from build123d import *

# Parameters (mm, degrees)
F1_DEPTH = 30
F0_W     = 30
F0_H     = 61.715728
F2_DEPTH = 60


with BuildPart() as f1:
    # F0 (on Front) → F1 (new body)
    with BuildSketch(Plane.XZ):
        with BuildLine():
            Line((-168.30257, -116.075176), (-168.30257, -201.93304))
            ThreePointArc((-168.30257, -201.93304), (-174.475736, -211.171836), (-185.373638, -209.004108))
            Line((-185.373638, -209.004108), (-265.373638, -129.004108))
            ThreePointArc((-265.373638, -129.004108), (-267.541366, -125.759875), (-268.30257, -121.93304))
            Line((-268.30257, -121.93304), (-298.30257, -121.93304))
            ThreePointArc((-298.30257, -121.93304), (-298.07544, -124.052242), (-297.404367, -126.075176))
            ThreePointArc((-297.404367, -126.075176), (-296.520542, -127.630843), (-295.373638, -129.004108))
            Line((-295.373638, -129.004108), (-171.231502, -253.146244))
            ThreePointArc((-171.231502, -253.146244), (-167.987269, -255.313971), (-164.160435, -256.075176))
            Line((-164.160435, -256.075176), (27.555294, -256.075176))
            ThreePointArc((27.555294, -256.075176), (31.382128, -255.313971), (34.626362, -253.146244))
            Line((34.626362, -253.146244), (158.768498, -129.004108))
            ThreePointArc((158.768498, -129.004108), (159.915401, -127.630843), (160.799227, -126.075176))
            ThreePointArc((160.799227, -126.075176), (161.4703, -124.052242), (161.69743, -121.93304))
            Line((161.69743, -121.93304), (131.69743, -121.93304))
            Line((131.69743, -121.93304), (131.69743, -60.217312))
            Line((131.69743, -60.217312), (161.69743, -60.217312))
            ThreePointArc((161.69743, -60.217312), (161.4703, -58.09811), (160.799227, -56.075176))
            ThreePointArc((160.799227, -56.075176), (159.915401, -54.51951), (158.768498, -53.146244))
            Line((158.768498, -53.146244), (33.456261, 72.165993))
            ThreePointArc((33.456261, 72.165993), (31.958527, 74.081905), (30.967545, 76.302689))
            Line((30.967545, 76.302689), (-43.30257, 318.264572))
            Line((-43.30257, 318.264572), (-93.30257, 318.264572))
            Line((-93.30257, 318.264572), (-167.572686, 76.302689))
            ThreePointArc((-167.572686, 76.302689), (-168.563667, 74.081905), (-170.061401, 72.165993))
            Line((-170.061401, 72.165993), (-295.373638, -53.146244))
            ThreePointArc((-295.373638, -53.146244), (-296.520542, -54.51951), (-297.404367, -56.075176))
            ThreePointArc((-297.404367, -56.075176), (-298.07544, -58.09811), (-298.30257, -60.217312))
            Line((-298.30257, -60.217312), (-268.30257, -60.217312))
            ThreePointArc((-268.30257, -60.217312), (-267.541366, -56.390477), (-265.373638, -53.146244))
            Line((-265.373638, -53.146244), (-171.231502, 40.995892))
            ThreePointArc((-171.231502, 40.995892), (-167.987269, 43.163619), (-164.160435, 43.924824))
            Line((-164.160435, 43.924824), (-103.30257, 43.924824))
            ThreePointArc((-103.30257, 43.924824), (-96.231502, 40.995892), (-93.30257, 33.924824))
            Line((-93.30257, 33.924824), (-93.30257, -96.075176))
            ThreePointArc((-93.30257, -96.075176), (-96.231502, -103.146244), (-103.30257, -106.075176))
            Line((-103.30257, -106.075176), (-158.30257, -106.075176))
            ThreePointArc((-158.30257, -106.075176), (-165.373638, -109.004108), (-168.30257, -116.075176))
        make_face()
        with BuildLine():
            Line((-2.753531, 73.924824), (-133.85161, 73.924824))
            ThreePointArc((-133.85161, 73.924824), (-141.893492, 77.981076), (-143.411393, 86.859196))
            Line((-143.411393, 86.859196), (-80.689379, 291.198944))
            ThreePointArc((-80.689379, 291.198944), (-77.073344, 296.306453), (-71.129596, 298.264572))
            Line((-71.129596, 298.264572), (-65.475545, 298.264572))
            ThreePointArc((-65.475545, 298.264572), (-59.531797, 296.306453), (-55.915761, 291.198944))
            Line((-55.915761, 291.198944), (6.806253, 86.859196))
            ThreePointArc((6.806253, 86.859196), (5.288351, 77.981076), (-2.753531, 73.924824))
        make_face(mode=Mode.SUBTRACT)
    extrude(amount=F1_DEPTH)

    # F0 (on Front) → F2 (join)
    with BuildSketch(Plane.XZ):
        with Locations((-283.30257, -91.075176)):
            Rectangle(F0_W, F0_H)
        with Locations((146.69743, -91.075176)):
            Rectangle(F0_W, F0_H)
    extrude(amount=F2_DEPTH)


solid = f1.part
The listing builds one solid part. Answer for the finished solid, in the listing's coordinates (mm). A direction names the side the tool comes from. Coordinates: 2 decimals unless noted, no trailing zeros. Loops run counter-clockwise (first coordinate to the right, second up) from the corner with the lowest first, then second, coordinate; pieces in that order, holes last. Notation, with made-up numbers: (68, -14) -> (76, -14) arc R22 cw to (76, 20) -> close; hole circle Ø11 at (72, 68.25). An arc over 180 degrees is marked (long way). Write item = value, one per line. Start each with the question number.
1) The mould has two halves that part along Z. Classify faces 1 (the face through (-224.814, -14.79, -169.564)), 2 (the face through (-284, -45, -60.217)), 3 (the face through (-35, -30, -53)): released by +Z, released by -Z, zero draft, split by the parting line, or undercut.
2) Given pin 1 Ø12 at (x, z) = (64, 44.5) entering from -Y; pin 2 Ø10 at (y, z) = (-26.5, -17) entering from +X; pin 3 Ø2 at (x, y) = (-214.5, -21) entering from +Z; pin 4 Ø4 at (x, y) = (-84.5, -33.5) entering from +Z, each flat-ended and moving along its own axis, determine where each tip first touches the part or whether it passes through.
3) A tool of negligible diameter and unlimited length cuts with its end or side. For faces 4 (the face through (96.99, -14.79, 8.63)), 5 (the face through (5.37, -14.79, 78.09)), from which of +Z, -Z, +X, -X, +Y, -Y can it reach the whole face along a straight path? Write none if from no direction.
4) A cutting plane is placed at B-B (z = -150). Give the vertices of the cut face in (x, y).
5) Straight lines are drawn through the part: line 1 (X direction, y = -35.5, z = -97.5); line 2 (X direction, y = -29.5, z = -88); line 3 (Y direction, x = 5.5, z = 98.5). For each, find the intervals that lie inside material, in ascending order. Write a range as from..to.
6) A cutting plane is placed at A-A (y = -52). Give the vertices of the cut face in (x, z).
7) A cutting plane is placed at D-D (x = 107). Give the vertices of the cut face in (y, z), then the cut area to 3 significant figures.
8) A cutting plane is placed at C-C (y = -21.5). Count the separate pieces of the cut face and the enclosed holes in it, then the cut area to 3 significant figures.
Responses:
q1.face_1 = undercut
q1.face_2 = released by +Z
q1.face_3 = zero draft
q2.pin_1 = -30
q2.pin_2 = 127.62
q2.pin_3 = 28.73
q2.pin_4 = through
q3.face_4 = +Z, +X, +Y, -Y
q3.face_5 = +Y, -Y
q4.outline = (-274.38, -30) -> (-244.38, -30) -> (-244.38, 0) -> (-274.38, 0) -> close; (-168.3, -30) -> (137.77, -30) -> (137.77, 0) -> (-168.3, 0) -> close
q5.line_1 = -298.3..-268.3, 131.7..161.7
q5.line_2 = -298.3..-268.3, -93.3..161.7
q5.line_3 = -30..0
q6.outline = (-298.3, -121.93) -> (-268.3, -121.93) -> (-268.3, -60.22) -> (-298.3, -60.22) -> close; (131.7, -121.93) -> (161.7, -121.93) -> (161.7, -60.22) -> (131.7, -60.22) -> close
q7.outline = (-30, -180.77) -> (0, -180.77) -> (0, -1.38) -> (-30, -1.38) -> close
q7.area = 5,380 mm²
q8.separate_pieces = 1
q8.enclosed_holes = 2
q8.area = 101,000 mm²
